from build123d import *

# Parameters (mm, degrees)
F1_DEPTH = 177.8
F3_DEPTH = 25.4


with BuildPart() as f1:
    # F0 (on Front) → F1 (new body)
    with BuildSketch(Plane.XZ):
        with BuildLine():
            ThreePointArc((0, 0.5), (0.146447, 0.146447), (0.5, 0))
            Line((0.5, 0), (101.1, 0))
            ThreePointArc((101.1, 0), (101.453553, 0.146447), (101.6, 0.5))
            Line((101.6, 0.5), (101.6, 4.5))
            ThreePointArc((101.6, 4.5), (101.453553, 4.853553), (101.1, 5))
            Line((101.1, 5), (98.1, 5))
            ThreePointArc((98.1, 5), (97.746447, 4.853553), (97.6, 4.5))
            Line((97.6, 4.5), (97.6, 3.2))
            ThreePointArc((97.6, 3.2), (97.541421, 3.058579), (97.4, 3))
            Line((97.4, 3), (70.88, 3))
            Line((70.88, 3), (65.8, 5))
            Line((65.8, 5), (35.8, 5))
            Line((35.8, 5), (30.72, 3))
            Line((30.72, 3), (4.2, 3))
            ThreePointArc((4.2, 3), (4.058579, 3.058579), (4, 3.2))
            Line((4, 3.2), (4, 4.5))
            ThreePointArc((4, 4.5), (3.853553, 4.853553), (3.5, 5))
            Line((3.5, 5), (0.5, 5))
            ThreePointArc((0.5, 5), (0.146447, 4.853553), (0, 4.5))
            Line((0, 4.5), (0, 0.5))
        make_face()
    extrude(amount=F1_DEPTH)

    # F2 (on face) → F3 (cut)
    with BuildSketch(Plane(origin=(0, 0, 0), x_dir=(-1, 0, 0), z_dir=(0, 1, 0))):
        with BuildLine():
            Line((0, 2.5), (-101.6, 2.5))
            Line((-101.6, 2.5), (-101.6, 0.5))
            ThreePointArc((-101.6, 0.5), (-101.453553, 0.146447), (-101.1, 0))
            Line((-101.1, 0), (-0.5, 0))
            ThreePointArc((-0.5, 0), (-0.146447, 0.146447), (0, 0.5))
            Line((0, 0.5), (0, 2.5))
        make_face()
    extrude(amount=-F3_DEPTH, mode=Mode.SUBTRACT)


solid = f1.part
Geometry check sheet. Reference: the model listing, model coordinates, mm. A direction names the side the tool comes from. Round coordinates to 2 decimals unless told otherwise and drop trailing zeros. Write each loop counter-clockwise with the first axis right and the second up, starting at its lowest first coordinate (ties: lowest second). Pieces come first, ordered by that corner, then holes. Notation, with made-up numbers: (28, 46) - (81, 46) arc R14 cw to (81, 64) - close; hole circle Ø7 at (60.25, 57). An arc over 180 degrees is marked (long way). One line per item, written item: value.
1. Cross-section at A-A on y = -11. Record the boundary of the cut face in (x, z), and give its area (3 significant figures).
The answers:
outline: (0, 2.5) - (101.6, 2.5) - (101.6, 4.5) arc R0.5 ccw to (101.1, 5) - (98.1, 5) arc R0.5 ccw to (97.6, 4.5) - (97.6, 3.2) arc R0.2 cw to (97.4, 3) - (70.88, 3) - (65.8, 5) - (35.8, 5) - (30.72, 3) - (4.2, 3) arc R0.2 cw to (4, 3.2) - (4, 4.5) arc R0.5 ccw to (3.5, 5) - (0.5, 5) arc R0.5 ccw to (0, 4.5) - close
area: 137 mm^2
2. Cross-section at D-D on z = 1.6. Record the boundary of the cut face in (x, y), and give its area (3 significant figures).
The answers:
outline: (0, -177.8) - (101.6, -177.8) - (101.6, -25.4) - (0, -25.4) - close
area: 15,500 mm^2
3. Scan lines: L1, parallel to Y at x = 74, z = 1.5; L2, parallel to Z at x = 96.5, y = -19; L3, parallel to Z at x = 88, y = -130. Record each from-to range of solid material in increasing order.
The answers:
L1: y = -177.8 to -25.4
L2: z = 2.5 to 3
L3: z = 0 to 3
4. Depth check by flat-ended pin: pin 1 Ø1.5 at (x, z) = (15.5, 1.5) entering from +Y; pin 2 Ø12.5 at (x, y) = (59, -18.5) entering from -Z. Enter the tip coordinate at first touch or a pass-through.
The answers:
pin 1: stops at y = -25.4
pin 2: stops at z = 2.5
5. Cross-section at B-B on x = 23. Record the boundary of the cut face in (y, z), and give its area (3 significant figures).
The answers:
outline: (-177.8, 0) - (-25.4, 0) - (-25.4, 2.5) - (0, 2.5) - (0, 3) - (-177.8, 3) - close
area: 470 mm^2
6. Cross-section at C-C on y = -52. Record the boundary of the cut face in (x, z), and give its area (3 significant figures).
The answers:
outline: (0, 0.5) arc R0.5 ccw to (0.5, 0) - (101.1, 0) arc R0.5 ccw to (101.6, 0.5) - (101.6, 4.5) arc R0.5 ccw to (101.1, 5) - (98.1, 5) arc R0.5 ccw to (97.6, 4.5) - (97.6, 3.2) arc R0.2 cw to (97.4, 3) - (70.88, 3) - (65.8, 5) - (35.8, 5) - (30.72, 3) - (4.2, 3) arc R0.2 cw to (4, 3.2) - (4, 4.5) arc R0.5 ccw to (3.5, 5) - (0.5, 5) arc R0.5 ccw to (0, 4.5) - close
area: 391 mm^2
7. Set-up check for faces 4 (the face through (84, -88, 3)), 5 (the face through (50, -13, 2.5)), 6 (the face through (50, -177.8, 2)): record each of +Z, -Z, +X, -X, +Y, -Y from which the full face is reachable in a straight line by a thin tool's end or side.
The answers:
face 4: +Z, +Y, -Y
face 5: -Z, +X, -X, +Y
face 6: +Z, -Z, +X, -X, -Y
8. Mould release check, pull along X, two halves, no side actions. Record for faces 1 (the face through (101.6, -88, 2)), 2 (the face through (0, -88, 3)), 3 (the face through (68.376, -87.655, 3.986)): released by +X, released by -X, zero draft, split by the parting line, or undercut.
The answers:
face 1: released by +X
face 2: released by -X
face 3: undercut
